```python
from build123d import *

# Parameters (mm, degrees)
MODEL_R             = 2.6
MODEL_R_2           = 1.25
MODEL_R_3           = 2.2
MODEL_R_4           = 2.1
MODEL_R_5           = 2.75
MODEL_R_6           = 1.5
MODEL_R_7           = 3.25
MODEL_R_8           = 26
BOSS_EXTRUDE1_DEPTH = 3
SKETCH1_R           = 2
CUT_EXTRUDE1_DEPTH  = 4


with BuildPart() as part:
    # Model → Boss-Extrude1 (new body)
    with BuildSketch(Plane.XY):
        Polygon((5, 150), (0, 150), (0, 50), (50, 0), (237, 0), (287, 50), (287, 150), (282, 150), (282, 138), (246.5, 138), (246.5, 150), (40.5, 150), (40.5, 138), (5, 138), align=None)
        with Locations((266.75, 125)):
            Circle(MODEL_R, mode=Mode.SUBTRACT)
        with Locations((261.75, 105)):
            Circle(MODEL_R, mode=Mode.SUBTRACT)
        with Locations((25.25, 105)):
            Circle(MODEL_R, mode=Mode.SUBTRACT)
        with Locations((20.25, 125)):
            Circle(MODEL_R, mode=Mode.SUBTRACT)
        with Locations((74.5, 96.7)):
            Circle(MODEL_R_2, mode=Mode.SUBTRACT)
        with Locations((93.5, 96.7)):
            Circle(MODEL_R_3, mode=Mode.SUBTRACT)
        with Locations((110, 60)):
            Circle(MODEL_R_4, mode=Mode.SUBTRACT)
        with Locations((77, 60)):
            Circle(MODEL_R_4, mode=Mode.SUBTRACT)
        with Locations((84.5, 60)):
            Circle(MODEL_R_2, mode=Mode.SUBTRACT)
        with Locations((102.5, 60)):
            Circle(MODEL_R_2, mode=Mode.SUBTRACT)
        with Locations((112.5, 96.7)):
            Circle(MODEL_R_2, mode=Mode.SUBTRACT)
        with Locations((193.5, 60)):
            Circle(MODEL_R_5, mode=Mode.SUBTRACT)
        with Locations((201.5, 60)):
            Circle(MODEL_R_6, mode=Mode.SUBTRACT)
        with Locations((185.5, 60)):
            Circle(MODEL_R_6, mode=Mode.SUBTRACT)
        with Locations((143.5, 23)):
            Circle(MODEL_R_7, mode=Mode.SUBTRACT)
        with Locations((193.5, 68)):
            Circle(MODEL_R_6, mode=Mode.SUBTRACT)
        with Locations((193.5, 52)):
            Circle(MODEL_R_6, mode=Mode.SUBTRACT)
        with Locations((237, 50)):
            Circle(MODEL_R_8, mode=Mode.SUBTRACT)
    extrude(amount=BOSS_EXTRUDE1_DEPTH)

    # Sketch1 → Cut-Extrude1 (cut, through all)
    with BuildSketch(Plane(origin=(0, 0, 0), x_dir=(-1, 0, 0), z_dir=(0, 0, -1))):
        with Locations((-202, 85)):
            Circle(SKETCH1_R)
        with Locations((-202, 15)):
            Circle(SKETCH1_R)
        with Locations((-272, 85)):
            Circle(SKETCH1_R)
    extrude(amount=-CUT_EXTRUDE1_DEPTH, mode=Mode.SUBTRACT)


solid = part.part
```
Input: part model. Units: mm. Frame: model coordinates. Coordinates: 2 decimals unless noted, no trailing zeros. Write each loop counter-clockwise with the first axis right and the second up, starting at its lowest first coordinate (ties: lowest second). Pieces come first, ordered by that corner, then holes. Notation, with made-up numbers: (-39.75, 23) -> (-17.75, 23) arc R18 cw to (-17.75, 41) -> close; hole circle Ø1 at (-9.5, -26). An arc over 180 degrees is marked (long way). Write each question's results on one line, items separated by ' | '.
Item 1: Section query A-A on x = 144. Return loops of the section in (y, z).
Conclusion:
outline: (0, 0) -> (19.79, 0) -> (19.79, 3) -> (0, 3) -> close; (26.21, 0) -> (150, 0) -> (150, 3) -> (26.21, 3) -> close
Item 2: Mould query, pull axis X, two halves, no side actions, for faces 1 (the cylindrical face through (24.912, 107.578, 1.479)), 2 (the flat face through (25, 25, 1)), 3 (the flat face through (141, 76, 3)). Classes: +X half, -X half, draft (parallel to the pull), parting line (faces both ways), or undercut.
Conclusion:
face 1: undercut | face 2: -X half | face 3: draft
Item 3: Section query B-B on z = 0.9. Count the separate pieces of the cut face and the enclosed holes in it, plus the area to 3 significant figures.
Conclusion:
separate pieces: 1 | enclosed holes: 21 | area: 37,300 mm^2
Item 4: Material intervals for probe 1 along Y at (x, z) = (193.5, 0.8); probe 2 along Y at (x, z) = (102.5, 1.2); probe 3 along X at (y, z) = (83.5, 2.3), sorted ascending.
Conclusion:
probe 1: y = 0 to 50.5, 53.5 to 57.25, 62.75 to 66.5, 69.5 to 150 | probe 2: y = 0 to 58.75, 61.25 to 150 | probe 3: x = 0 to 200.68, 203.32 to 270.68, 273.32 to 287
